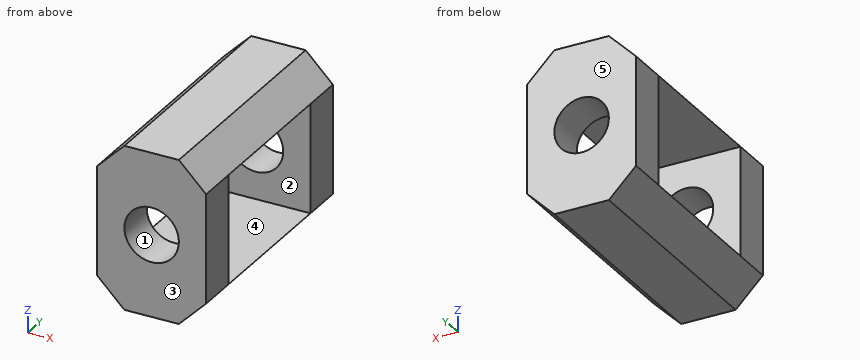
```python
from build123d import *

# Parameters (mm, degrees)
SKETCH1_W           = 8
SKETCH1_H           = 12
SKETCH1_R           = 2
BOSS_EXTRUDE1_DEPTH = 17
SKETCH2_W           = 8
SKETCH2_H           = 11
CUT_EXTRUDE1_DEPTH  = 17
CHAMFER1_SIZE       = 2


with BuildPart() as part:
    # Sketch1 → Boss-Extrude1 (new body)
    with BuildSketch(Plane(origin=(0, 0, 0), x_dir=(1, 0, 0), z_dir=(0, 1, 0))):
        Rectangle(SKETCH1_W, SKETCH1_H)
        with Locations(Location((0, 0, 0), (0, 0, 270))):
            Circle(SKETCH1_R, mode=Mode.SUBTRACT)
    extrude(amount=BOSS_EXTRUDE1_DEPTH)

    # Sketch2 → Cut-Extrude1 (cut)
    with BuildSketch(Plane(origin=(4, 0, 0), x_dir=(0, 0, -1), z_dir=(1, 0, 0))):
        with Locations((0, 8.5)):
            Rectangle(SKETCH2_W, SKETCH2_H)
    extrude(amount=-CUT_EXTRUDE1_DEPTH, mode=Mode.SUBTRACT)

    # Chamfer1
    chamfer1_edges = [part.edges().sort_by_distance(p)[0] for p in [
        (4, 8.5, 6),
        (-4, 8.5, 6),
        (-4, 8.5, -6),
        (4, 8.5, -6),
    ]]
    chamfer(chamfer1_edges, length=CHAMFER1_SIZE - 0.0001)  # a hair under: the kernel refuses the full size


solid = part.part
```
Check sheet for the modelled part. Datum: model origin and axes. Units: mm. Face numbers are marked on the shaded views. A direction names the side the tool comes from. Give positions to 0.01 mm unless a question says otherwise; leave off trailing zeros. Write each loop counter-clockwise with the first axis right and the second up, starting at its lowest first coordinate (ties: lowest second). Pieces come first, ordered by that corner, then holes. Notation, with made-up numbers: (88.25, 62.5) -> (114.25, 62.5) arc R24 cw to (114.25, 80.5) -> close; hole circle Ø11 at (89.25, -2). An arc over 180 degrees is marked (long way). Use CSV: the item, a comma, the result in double quotes. Start each with the question number.
Q1. Scan lines: line 1 along Z through (x, y) = (1.25, 5.75); line 2 along X through (y, z) = (0.95, 0); line 3 along Z through (x, y) = (0, 1.15). Record each from-to range of solid material in increasing order.
Q2. Tool access check on the marked faces 4 and 5. Record the directions out of +Z, -Z, +X, -X, +Y, -Y that give a thin tool (end or side, any length) a straight path to the whole face; none if there is none.
Q3. Cross-section at B-B on z = 0. Enter the section's corners in (x, y), and give its area (3 significant figures).
Q4. Cross-section at C-C on x = 0. Enter the section's corners in (y, z).
Q5. Cross-section at A-A on z = 3.75. Enter the section's corners in (x, y), and give its area (3 significant figures).
Q6. Release check for a two-part mould opening along Y. For the marked faces 1, 2 and 3 record: +Y half, -Y half, draft (parallel to the pull), parting line (faces both ways), or undercut.
Working result:
1,line 1,"z = -6 to -4, 4 to 6"
1,line 2,"x = -4 to -2, 2 to 4"
1,line 3,"z = -6 to -2, 2 to 6"
2,face 4,"+X, -X"
2,face 5,"+Z, -Z, +X, -X, +Y"
3,outline,"(-4, 0) -> (-2, 0) -> (-2, 3) -> (-4, 3) -> close; (-4, 14) -> (-2, 14) -> (-2, 17) -> (-4, 17) -> close; (2, 0) -> (4, 0) -> (4, 3) -> (2, 3) -> close; (2, 14) -> (4, 14) -> (4, 17) -> (2, 17) -> close"
3,area,"24.0 mm^2"
4,outline,"(0, -6) -> (17, -6) -> (17, -2) -> (14, -2) -> (14, -4) -> (3, -4) -> (3, -2) -> (0, -2) -> close; (0, 2) -> (3, 2) -> (3, 4) -> (14, 4) -> (14, 2) -> (17, 2) -> (17, 6) -> (0, 6) -> close"
5,outline,"(-4, 0) -> (4, 0) -> (4, 3) -> (-4, 3) -> close; (-4, 14) -> (4, 14) -> (4, 17) -> (-4, 17) -> close"
5,area,"48.0 mm^2"
6,face 1,"draft"
6,face 2,"undercut"
6,face 3,"-Y half"
